Part print with two shaded views. Sizes in mm from the minimum x, y, z corner. A direction names the side the tool comes from. Coordinates: 2 decimals unless noted, no trailing zeros. Loops run counter-clockwise (first coordinate to the right, second up) from the corner with the lowest first, then second, coordinate; pieces in that order, holes last. Notation, with made-up numbers: (26.25, 46.5) -> (47.25, 46.5) arc R4 cw to (47.25, 51.5) -> close; hole circle Ø6 at (88, 59.25). An arc over 180 degrees is marked (long way). Write each question's results on one line, items separated by ' | '.
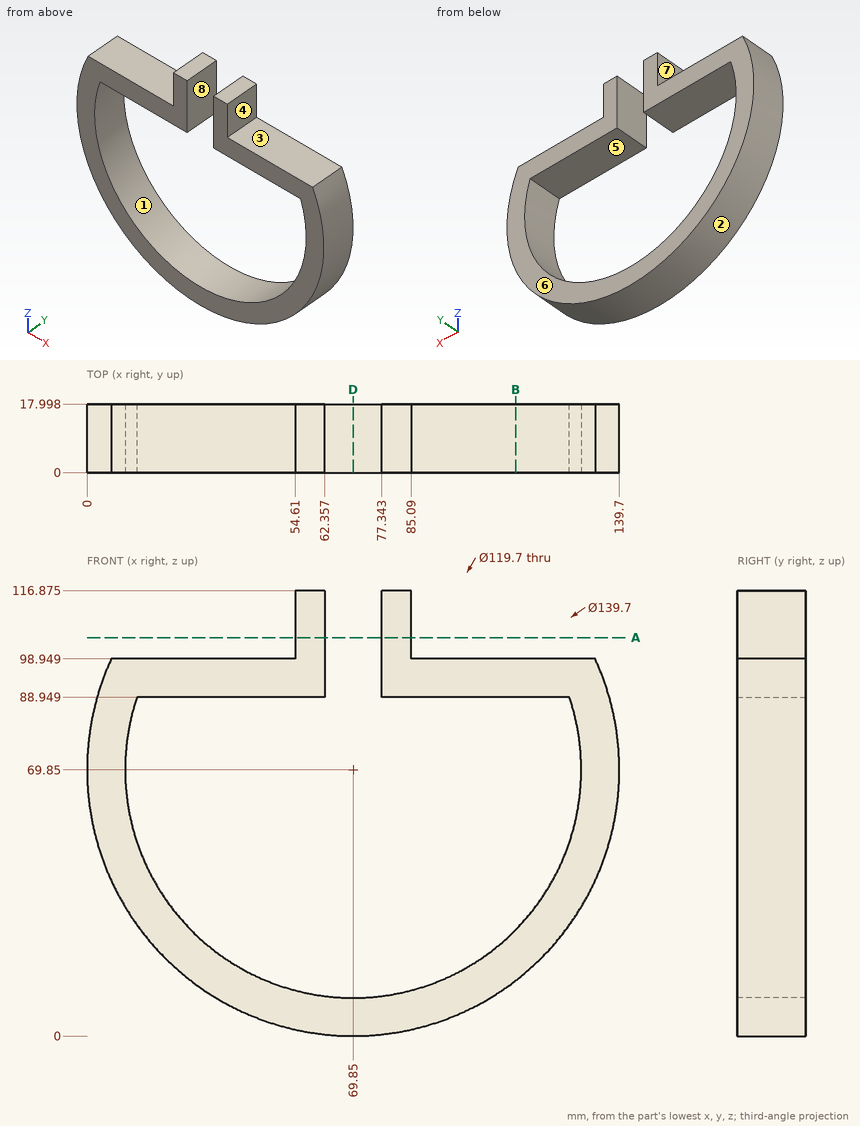
Q1. Pull direction X, two halves, no side cores. Call the marked faces 1, 2 and 3: +X half, -X half, draft (parallel to the pull), parting line (faces both ways), or undercut.
Results are:
face 1: undercut | face 2: parting line | face 3: draft
Q2. Wall check: L1, parallel to X at y = 1, z = 111; L2, parallel to X at y = 13, z = 69.85; L3, parallel to Z at x = 70, y = 2.75. Give the ranges that are in metal, low to high. Write a range as from..to.
Results are:
L1: 54.61..62.36, 77.34..85.09 | L2: 0..10, 129.7..139.7 | L3: 0..10
Q3. Cut at D-D on x = 69.85. Write the cut outline in (y, z).
Results are:
outline: (0, 0) -> (18, 0) -> (18, 10) -> (0, 10) -> close
Q4. Drop flat-ended pins along their axis: pin 1 (2 mm diameter, centred on y = 5.5, z = 13.5, fed in from +X); pin 2 (1.5 mm diameter, centred on x = 64, z = 98, fed in from +Y); pin 3 (5.5 mm diameter, centred on y = 9, z = 101, fed in from +X) (1 decimal); pin 4 (9 mm diameter, centred on x = 95, y = 13.5, fed in from -Z). Give the stop position or say it passes through.
Results are:
pin 1: x = 112.46 | pin 2: through | pin 3: x = 133.7 | pin 4: z = 3.12
Q5. Cut at A-A on z = 104.5. Write the cut outline in (x, y), and give its area (3 significant figures).
Results are:
outline: (54.61, 0) -> (62.36, 0) -> (62.36, 18) -> (54.61, 18) -> close; (77.34, 0) -> (85.09, 0) -> (85.09, 18) -> (77.34, 18) -> close | area: 279 mm^2
Q6. Cut at B-B on x = 112.5. Write the cut outline in (y, z).
Results are:
outline: (0, 14.53) -> (18, 14.53) -> (18, 27.86) -> (0, 27.86) -> close; (0, 88.95) -> (18, 88.95) -> (18, 98.95) -> (0, 98.95) -> close
Q7. Which spindle directions (+Z, -Z, +X, -X, +Y, -Y) get a long thin tool onto all of the face, cutting with end or side? Do the marked faces 4, 5, 6, 7 and 8. Say none if no direction does.
Results are:
face 4: +Z, +X, +Y, -Y | face 5: +Y, -Y | face 6: +Z, -Z, +X, -X, +Y | face 7: +Z, -X, +Y, -Y | face 8: +Z, +Y, -Y
